Verification items for this drawing (mm, ordinates from the low corner). A direction names the side the tool comes from. Give positions to 0.01 mm unless a question says otherwise; leave off trailing zeros. Write each loop counter-clockwise with the first axis right and the second up, starting at its lowest first coordinate (ties: lowest second). Pieces come first, ordered by that corner, then holes. Notation, with made-up numbers: (77.5, 0) -> (116.5, 0) arc R21 ccw to (116.5, 13) -> close; hole circle Ø1 at (-5.5, 15.25). An arc over 180 degrees is marked (long way). Write item = value, one per line.
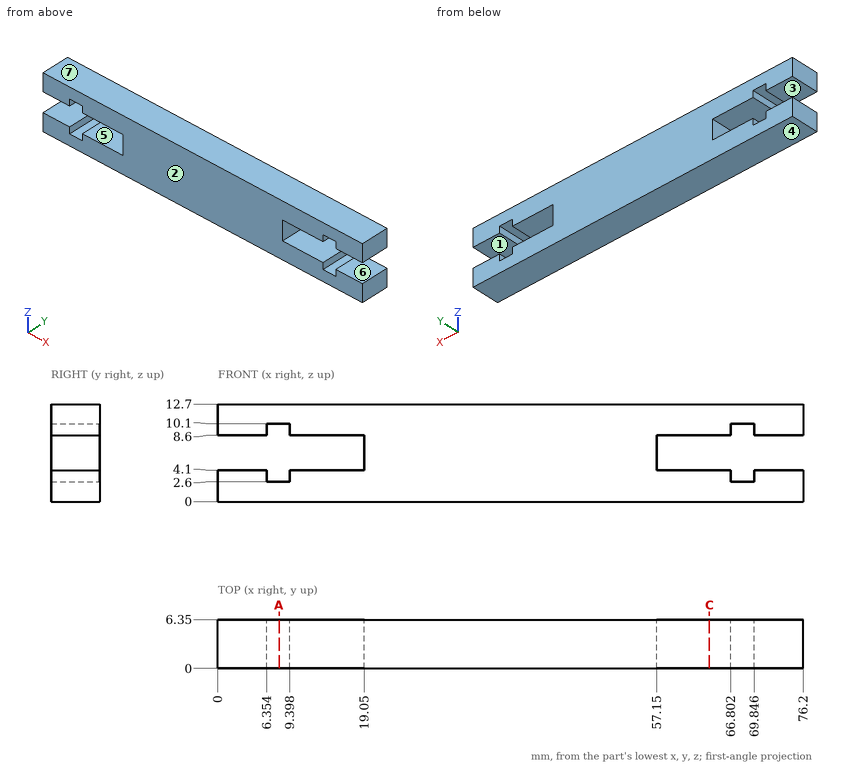
Item 1: Sectioned sample at C-C on x = 64. Record the cut outline in (y, z).
Response values:
outline = (0, 0) -> (6.35, 0) -> (6.35, 4.1) -> (0, 4.1) -> close; (0, 8.6) -> (6.35, 8.6) -> (6.35, 12.7) -> (0, 12.7) -> close
Item 2: Sectioned sample at A-A on x = 8. Record the cut outline in (y, z).
Response values:
outline = (0, 0) -> (6.35, 0) -> (6.35, 2.6) -> (0, 2.6) -> close; (0, 10.1) -> (6.35, 10.1) -> (6.35, 12.7) -> (0, 12.7) -> close
Item 3: Mould release check, pull along Z, two halves, no side actions. Record for the marked faces 4, 5, 6 and 7: +Z half, -Z half, draft (parallel to the pull), parting line (faces both ways), or undercut.
Response values:
face_4 = -Z half
face_5 = undercut
face_6 = undercut
face_7 = +Z half
Item 4: Go/stop test with a flat-tipped pin: P1, Ø1.5, axis at x = 68, y = 1.5, coming from the -Z side. Record where the tip stops, or that it passes through.
Response values:
P1 = 0
Item 5: Set-up check for the marked faces 1, 2 and 3: record each of +Z, -Z, +X, -X, +Y, -Y from which the full face is reachable in a straight line by a thin tool's end or side.
Response values:
face_1 = +X, +Y, -Y
face_2 = +Z, -Z, +X, -X, -Y
face_3 = -X, +Y, -Y
Item 6: Material ranges on line 1 (X direction, y = 3, z = 9) (1 decimal); line 2 (Z direction, x = 73.5, y = 3); line 3 (Z direction, x = 9, y = 1.75), recorded low to high.
Response values:
line_1 = 0 to 6.4, 9.4 to 66.8, 69.8 to 76.2
line_2 = 0 to 4.1, 8.6 to 12.7
line_3 = 0 to 2.6, 10.1 to 12.7
